Verification items for the finished model (mm, model axes). A direction names the side the tool comes from. Round coordinates to 2 decimals unless told otherwise and drop trailing zeros. Write each loop counter-clockwise with the first axis right and the second up, starting at its lowest first coordinate (ties: lowest second). Pieces come first, ordered by that corner, then holes. Notation, with made-up numbers: M 74.25,42.25 L 100.25,42.25 A25 ccw 100.25,70.25 Z; hole C -17.5,32.5 d1. An arc over 180 degrees is marked long. Write each question's results on one line, items separated by ' | '.
from build123d import *

# Parameters (mm, degrees)
SKETCH1_R           = 55.5625
BOSS_EXTRUDE1_DEPTH = 76.2
SKETCH2_R           = 52.3875
CUT_EXTRUDE1_DEPTH  = 31.75
CUT_EXTRUDE1_TAPER  = 37
SKETCH3_R           = 52.3875
CUT_EXTRUDE2_DEPTH  = 31.75
CUT_EXTRUDE2_TAPER  = 37
SKETCH4_R           = 18.5
SKETCH4_R_2         = 17
BOSS_EXTRUDE2_DEPTH = 44.45


with BuildPart() as part:
    # Sketch1 → Boss-Extrude1 (new body)
    with BuildSketch(Plane(origin=(0, 0, 0), x_dir=(0, 0, -1), z_dir=(1, 0, 0))):
        Circle(SKETCH1_R)
    extrude(amount=BOSS_EXTRUDE1_DEPTH)

    # Sketch2 → Cut-Extrude1 (cut)
    with BuildSketch(Plane(origin=(76.2, 0, 0), x_dir=(0, 0, -1), z_dir=(1, 0, 0))):
        Circle(SKETCH2_R)
    extrude(amount=-CUT_EXTRUDE1_DEPTH, taper=CUT_EXTRUDE1_TAPER, mode=Mode.SUBTRACT)

    # Sketch3 → Cut-Extrude2 (cut)
    with BuildSketch(Plane.ZY):
        Circle(SKETCH3_R)
    extrude(amount=-CUT_EXTRUDE2_DEPTH, taper=CUT_EXTRUDE2_TAPER, mode=Mode.SUBTRACT)

    # Sketch4 → Boss-Extrude2 (add)
    with BuildSketch(Plane(origin=(44.45, 0, 0), x_dir=(0, 0, -1), z_dir=(1, 0, 0))):
        Circle(SKETCH4_R)
        Circle(SKETCH4_R_2, mode=Mode.SUBTRACT)
    extrude(amount=BOSS_EXTRUDE2_DEPTH)


solid = part.part
1) Depth check by flat-ended pin: P1, Ø10, axis at y = 31, z = -31, coming from the -X side; P2, Ø1, axis at x = 38, z = 32.5, coming from the +Y side; P3, Ø1.5, axis at x = 73.5, z = -1, coming from the +Y side. Enter the tip coordinate at first touch or a pass-through.
Calculated:
P1: stops at x = 4.71 | P2: stops at y = 45.42 | P3: stops at y = 55.56
2) Sectioned sample at A-A, the plane z = 0. Record the cut outline in (x, y).
Calculated:
outline: M 0,-55.56 L 76.2,-55.56 L 76.2,-52.39 L 44.45,-28.46 L 44.45,-18.5 L 88.9,-18.5 L 88.9,-17 L 44.45,-17 L 44.45,17 L 88.9,17 L 88.9,18.5 L 44.45,18.5 L 44.45,28.46 L 76.2,52.39 L 76.2,55.56 L 0,55.56 L 0,52.39 L 31.75,28.46 L 31.75,-28.46 L 0,-52.39 Z
3) Draft check along Y on faces 4 (the flat face through (0, 17, 50)), 5 (the cylindrical face through (66.36, -18.06, 4.01)), 6 (the conical face through (45.992, 8.898, -28.256)), 7 (the cylindrical face through (37.57, 55.09, 7.23)). Enter one of: pulls with the +Y half, pulls with the -Y half, needs draft (parallel to the pull), parting line crosses it, or undercut.
Calculated:
face 4: needs draft | face 5: undercut | face 6: undercut | face 7: parting line crosses it
4) Access from +Z, -Z, +X, -X, +Y, -Y to the whole of each face (thin tool, end or side, straight path). Record for faces 1 (the flat face through (31.75, 0, 0)), 2 (the flat face through (88.9, -16.4, -5.4)), 3 (the flat face through (44.45, 0, 0)).
Calculated:
face 1: -X | face 2: +Z, -Z, +X, +Y, -Y | face 3: +X
5) Sectioned sample at C-C, the plane x = 34. Record the cut outline in (y, z) (1 decimal).
Calculated:
outline: C 0,0 d111.1
6) Material ranges on line 1 (Z direction, x = 50, y = -6); line 2 (Z direction, x = 63.5, y = -11); line 3 (Y direction, x = 66, z = 0), recorded low to high. Write a range as [from, to].
Calculated:
line 1: z = [-55.24, -32.09], [-17.5, -15.91], [15.91, 17.5], [32.09, 55.24] | line 2: z = [-54.46, -41.38], [-14.87, -12.96], [12.96, 14.87], [41.38, 54.46] | line 3: y = [-55.56, -44.7], [-18.5, -17], [17, 18.5], [44.7, 55.56]
7) Sectioned sample at D-D, the plane x = 47. Record the cut outline in (y, z) (1 decimal).
Calculated:
outline: C 0,0 d111.1; C 0,0 d37; hole C 0,0 d60.8; hole C 0,0 d34
8) Sectioned sample at B-B, the plane x = 68. Record the cut outline in (y, z) (1 decimal).
Calculated:
outline: C 0,0 d111.1; C 0,0 d37; hole C 0,0 d92.4; hole C 0,0 d34
